Build history of the part. All positions in model axes, mm. A direction names the side the tool comes from. Round coordinates to 2 decimals unless told otherwise and drop trailing zeros. Order: outer loops, then holes, each group sorted by start corner. A loop starts at its lowest first (then second) coordinate and runs counter-clockwise, first axis right, second up. Notation, with made-up numbers: (85, 14.25) -> (100, 14.25) arc R22 ccw to (100, 29.25) -> close; hole circle Ø3 at (-8, 59). An arc over 180 degrees is marked (long way). Use a Markdown table: item, result. Add a question column.
Item 1: Two-plate mould, pull along X, no slides. Class faces 4 (the face through (2, 1.406, 1)), 5 (the face through (1, 15, 0)), 6 (the face through (-6, 9, 0)): released by +X, released by -X, zero draft, split by the parting line, or undercut.
Item 2: Slice it at C-C, the plane y = 8. Give the cut face in (x, z), plus the area to 3 significant figures.
Item 3: Probe L1, parallel to Y at x = -0.75, z = -3.5; L2, parallel to X at y = 14.75, z = -0.5; L3, parallel to Y at x = -0.5, z = -1. List the from-to ranges inside material, lowest first.
Item 4: 3-axis set-ups, long thin cutter, end or side, ignore diameter. For faces 1 (the face through (0, 0.406, 0)), 2 (the face through (-1, 15, 0)), 3 (the face through (1.42, 8.406, 3.92)): which of +Z, -Z, +X, -X, +Y, -Y reach the whole face in a straight line?
Item 5: Pin check, flat tips, straight feed: pin 1 (4 mm diameter, centred on x = -3.5, y = 11.5, fed in from +Z); pin 2 (6 mm diameter, centred on x = 4, y = 4, fed in from +Z); pin 3 (1 mm diameter, centred on y = 16, z = 1, fed in from +X). Stop position of each tip, or through.
from build123d import *

# Parameters (mm, degrees)
SKETCH2_W          = 2
SKETCH2_H          = 4
CUT_EXTRUDE1_DEPTH = 5


with BuildPart() as part:
    # Sketch1 → Revolve1 (revolve)
    with BuildSketch(Plane.XY):
        with BuildLine():
            Line((6, 10.406467745), (5.997713172, 10.406467745))
            ThreePointArc((5.997713172, 10.406467745), (4.300804682, 14.755776187), (0, 16.572108049))
            Line((0, 16.572108049), (0, 0.406467745))
            Line((0, 0.406467745), (2, 0.406467745))
            Line((2, 0.406467745), (2, 1.406467745))
            Line((2, 1.406467745), (4, 1.406467745))
            Line((4, 1.406467745), (4, 8.406467745))
            Line((4, 8.406467745), (6, 8.406467745))
            Line((6, 8.406467745), (6, 10.406467745))
        make_face()
    revolve(axis=Axis((0, 0.406467745, 0), (0, 1, 0)))

    # Sketch2 → Cut-Extrude1 (cut, symmetric)
    with BuildSketch(Plane.XY):
        with Locations((0, 16.572108049)):
            Rectangle(SKETCH2_W, SKETCH2_H)
    extrude(amount=CUT_EXTRUDE1_DEPTH, both=True, mode=Mode.SUBTRACT)


solid = part.part
Check sheet entries:
| question | item | result |
|---|---|---|
| 1 | face 4 | zero draft |
| 1 | face 5 | undercut |
| 1 | face 6 | split by the parting line |
| 2 | outline | circle Ø8 at (0, 0) |
| 2 | area | 50.3 mm2 |
| 3 | L1 | 1.41 to 14.57 |
| 3 | L2 | -4.28 to -1, 1 to 4.28 |
| 3 | L3 | 0.41 to 14.57 |
| 4 | face 1 | +Z, -Z, +X, -X, -Y |
| 4 | face 2 | +Z, -Z, +Y |
| 4 | face 3 | -Y |
| 5 | pin 1 | z = 5.78 |
| 5 | pin 2 | z = 3.87 |
| 5 | pin 3 | x = 3.29 |
